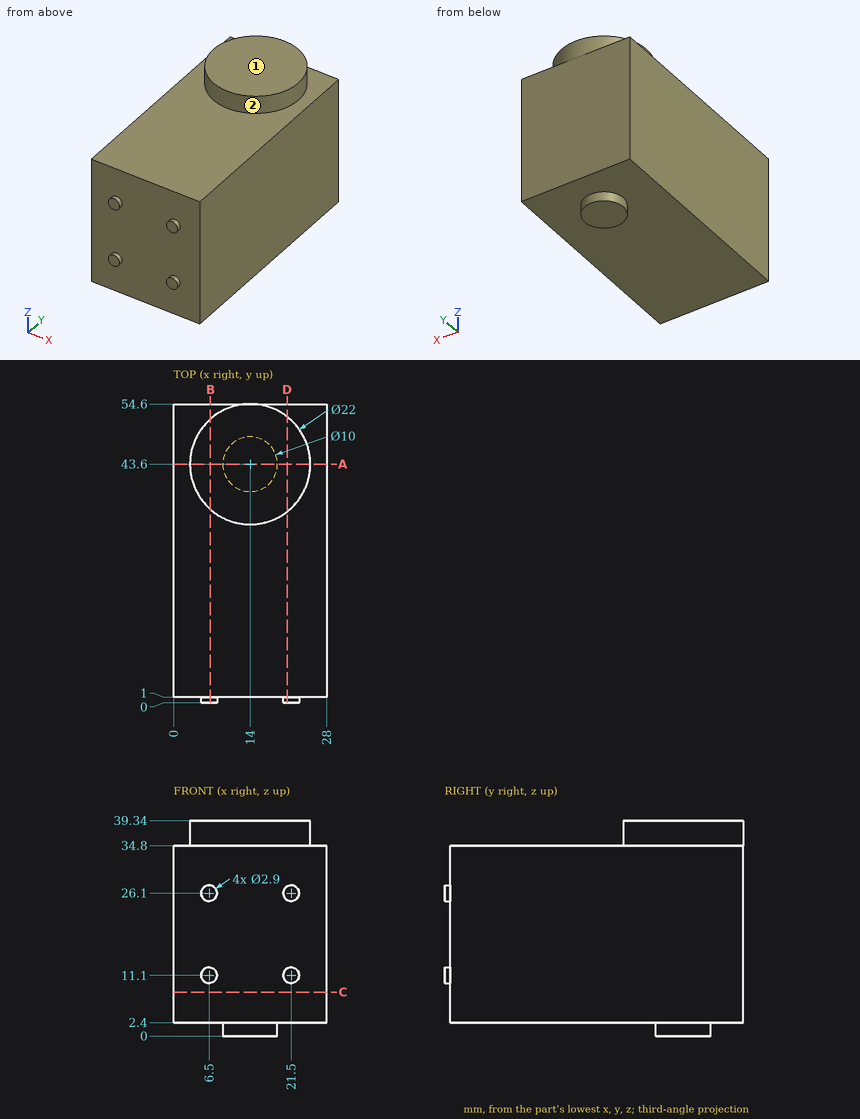
Design review of the part shown in the three views and the two pictorial views. Dimensions are in mm from the part's minimum x, y and z. A direction names the side the tool comes from. Coordinates: 2 decimals unless noted, no trailing zeros. Write each loop counter-clockwise with the first axis right and the second up, starting at its lowest first coordinate (ties: lowest second). Pieces come first, ordered by that corner, then holes. Notation, with made-up numbers: (46, -19.5) - (74, -19.5) arc R18 ccw to (74, 7.5) - close; hole circle Ø7 at (87, 48.5). An arc over 180 degrees is marked (long way). Write item = value, one per line.
(1) Consider section D-D, the plane x = 20.75. Give the boundary of the cut face in (y, z).
Result sheet:
outline = (0, 9.86) - (1, 9.86) - (1, 2.4) - (54.6, 2.4) - (54.6, 34.8) - (52.29, 34.8) - (52.29, 39.34) - (34.91, 39.34) - (34.91, 34.8) - (1, 34.8) - (1, 27.34) - (0, 27.34) - (0, 24.86) - (1, 24.86) - (1, 12.34) - (0, 12.34) - close
(2) Consider section A-A, the plane y = 43.6. Give the boundary of the cut face in (x, z), then the cut area to 3 significant figures.
Result sheet:
outline = (0, 2.4) - (9, 2.4) - (9, 0) - (19, 0) - (19, 2.4) - (28, 2.4) - (28, 34.8) - (25, 34.8) - (25, 39.34) - (3, 39.34) - (3, 34.8) - (0, 34.8) - close
area = 1,030 mm^2
(3) For line 1 (Z direction, x = 20.5, y = 47); line 2 (Z direction, x = 4.5, y = 8); line 3 (Y direction, x = 2.5, z = 20), list the stretches that pass through material, from the lowest coordinate up. Write a range as [from, to].
Result sheet:
line_1 = [2.4, 39.34]
line_2 = [2.4, 34.8]
line_3 = [1, 54.6]
(4) Consider section B-B, the plane x = 6.75. Give the boundary of the cut face in (y, z), then the cut area to 3 significant figures.
Result sheet:
outline = (0, 9.67) - (1, 9.67) - (1, 2.4) - (54.6, 2.4) - (54.6, 34.8) - (51.87, 34.8) - (51.87, 39.34) - (35.33, 39.34) - (35.33, 34.8) - (1, 34.8) - (1, 27.53) - (0, 27.53) - (0, 24.67) - (1, 24.67) - (1, 12.53) - (0, 12.53) - close
area = 1,820 mm^2
(5) Machinability: for the marked faces 1 and 2, which of the approach directions +Z, -Z, +X, -X, +Y, -Y give a long, thin tool a straight path to every point of the face, cutting with its end or side? Answer none if there is none.
Result sheet:
face_1 = +Z, +X, -X, +Y, -Y
face_2 = +Z
(6) Consider section C-C, the plane z = 8. Give the boundary of the cut face in (x, y), then the cut area to 3 significant figures.
Result sheet:
outline = (0, 1) - (28, 1) - (28, 54.6) - (0, 54.6) - close
area = 1,500 mm^2
(7) For P1, Ø6, axis at x = 8, y = 32.5, coming from the -Z side; P2, Ø5, axis at y = 35, z = 8.5, coming from the -X side; P3, Ø4, axis at x = 7, y = 22.5, coming from the +Z side, all flat-tipped, find the tip position at first contact; note any pin that passes through.
Result sheet:
P1 = 2.4
P2 = 0
P3 = 34.8
